Geometry: final body of the model. Coordinates: model frame, mm. A direction names the side the tool comes from. Give positions to 0.01 mm unless a question says otherwise; leave off trailing zeros. Order: outer loops, then holes, each group sorted by start corner. A loop starts at its lowest first (then second) coordinate and runs counter-clockwise, first axis right, second up. Notation, with made-up numbers: M 10.25,-24.5 L 15.25,-24.5 A35 ccw 15.25,11.5 Z; hole C 33,-27 d7. An arc over 180 degrees is marked long. Write item = value, one per line. Start each with the question number.
from build123d import *

# Parameters (mm, degrees)
IZIM1_R                     = 1.5
Y_KSEKLIK_EKSTR_ZYON1_DEPTH = 2
Y_KSEKLIK_EKSTR_ZYON2_START = -10
Y_KSEKLIK_EKSTR_ZYON2_DEPTH = 10
Y_KSEKLIK_EKSTR_ZYON3_START = -10
Y_KSEKLIK_EKSTR_ZYON3_DEPTH = 10
KAT_Y_D_N_T_R2_START        = 12.5
KAT_Y_D_N_T_R2_OUTLINE_W    = 10
KAT_Y_D_N_T_R2_OUTLINE_H    = 6
KAT_Y_D_N_T_R2_DEPTH        = 8
KAT_Y_D_N_T_R2_START_2      = 16.5
KAT_Y_D_N_T_R2_2_OUTLINE_W  = 10
KAT_Y_D_N_T_R2_2_OUTLINE_H  = 4
KAT_Y_D_N_T_R2_2_DEPTH      = 4
KENAR_START                 = -29.083147129
KENAR_EKME1_DEPTH           = 10
KENAR_START_2               = 19
KENAR_EKME1_2_DEPTH         = 10
PAH3_SIZE                   = 1


# Read off the part's stored shape, not the designer's step: Katıyı-Dönüştür2, Kenar Çekme1
with BuildPart() as part:
    # Çizim1 → Yükseklik-Ekstrüzyon1 (new body)
    with BuildSketch(Plane(origin=(0, 0, 0), x_dir=(1, 0, 0), z_dir=(0, 1, 0))):
        with BuildLine():
            Line((29, -12.5), (19, -12.5))
            Line((19, -12.5), (19, -6.464101615))
            Line((19, -6.464101615), (19, 3.5))
            ThreePointArc((19, 3.5), (18.121320344, 5.621320344), (16, 6.5))
            Line((16, 6.5), (-3.464101615, 6.5))
            Line((-3.464101615, 6.5), (-16.083147129, 6.5))
            ThreePointArc((-16.083147129, 6.5), (-18.204467472, 5.621320344), (-19.083147129, 3.5))
            Line((-19.083147129, 3.5), (-19.083147129, -6.464101615))
            Line((-19.083147129, -6.464101615), (-19.083147129, -12.5))
            Line((-19.083147129, -12.5), (-29.083147129, -12.5))
            Line((-29.083147129, -12.5), (-29.083147129, 13.5))
            ThreePointArc((-29.083147129, 13.5), (-28.204467472, 15.621320344), (-26.083147129, 16.5))
            Line((-26.083147129, 16.5), (26, 16.5))
            ThreePointArc((26, 16.5), (28.121320344, 15.621320344), (29, 13.5))
            Line((29, 13.5), (29, -12.5))
        make_face()
        with Locations(Location((-24.083147129, -3, 0), (0, 0, 270))):
            Circle(IZIM1_R, mode=Mode.SUBTRACT)
        with Locations(Location((0, 11.5, 0), (0, 0, 270))):
            Circle(IZIM1_R, mode=Mode.SUBTRACT)
        with Locations(Location((24, -3, 0), (0, 0, 270))):
            Circle(IZIM1_R, mode=Mode.SUBTRACT)
    extrude(amount=Y_KSEKLIK_EKSTR_ZYON1_DEPTH)

    # Çizim2 → Yükseklik-Ekstrüzyon2 (add)
    with BuildSketch(Plane(origin=(29, 0, 0), x_dir=(0, 0, -1), z_dir=(1, 0, 0)).offset(Y_KSEKLIK_EKSTR_ZYON2_START)):
        with BuildLine():
            Line((-14.767949192, 3), (-12.627016654, 3))
            ThreePointArc((-12.627016654, 3), (-18.949489743, 7.16227766), (-16.5, 0))
            Line((-16.5, 0), (-12.5, 0))
            Line((-12.5, 0), (-12.5, 2))
            Line((-12.5, 2), (-16.5, 2))
            ThreePointArc((-16.5, 2), (-17.5, 5.732050808), (-14.767949192, 3))
        make_face()
    extrude(amount=Y_KSEKLIK_EKSTR_ZYON2_DEPTH)

    # Çizim3 → Yükseklik-Ekstrüzyon3 (add)
    with BuildSketch(Plane(origin=(-19.083147129, 0, 0), x_dir=(0, 0, -1), z_dir=(1, 0, 0)).offset(Y_KSEKLIK_EKSTR_ZYON3_START)):
        with BuildLine():
            Line((-12.5, 2), (-16.5, 2))
            ThreePointArc((-16.5, 2), (-17.5, 5.732050808), (-14.767949192, 3))
            Line((-14.767949192, 3), (-12.627016654, 3))
            ThreePointArc((-12.627016654, 3), (-18.949489743, 7.16227766), (-16.5, 0))
            Line((-16.5, 0), (-12.5, 0))
            Line((-12.5, 0), (-12.5, 2))
        make_face()
    extrude(amount=Y_KSEKLIK_EKSTR_ZYON3_DEPTH)

    # Katıyı-Dönüştür2 outline → Katıyı-Dönüştür2 (cut)
    with BuildSketch(Plane.XY.offset(KAT_Y_D_N_T_R2_START)):
        with Locations((24, 6)):
            Rectangle(KAT_Y_D_N_T_R2_OUTLINE_W, KAT_Y_D_N_T_R2_OUTLINE_H)
        with Locations((-24.083147129, 6)):
            Rectangle(KAT_Y_D_N_T_R2_OUTLINE_W, KAT_Y_D_N_T_R2_OUTLINE_H)
    extrude(amount=KAT_Y_D_N_T_R2_DEPTH, mode=Mode.SUBTRACT)

    # Kat_y_-D_n_t_r2 2 outline → Kat_y_-D_n_t_r2 2 (cut)
    with BuildSketch(Plane.XY.offset(KAT_Y_D_N_T_R2_START_2)):
        with Locations((24, 1)):
            Rectangle(KAT_Y_D_N_T_R2_2_OUTLINE_W, KAT_Y_D_N_T_R2_2_OUTLINE_H)
        with Locations((-24.083147129, 1)):
            Rectangle(KAT_Y_D_N_T_R2_2_OUTLINE_W, KAT_Y_D_N_T_R2_2_OUTLINE_H)
    extrude(amount=KAT_Y_D_N_T_R2_2_DEPTH, mode=Mode.SUBTRACT)

    # Kenar Çekme1 outline → Kenar Çekme1 (add)
    with BuildSketch(Plane.YZ.offset(KENAR_START)):
        with BuildLine():
            Line((3.448725288, 14.577476608), (2.897450577, 12.654953216))
            ThreePointArc((2.897450577, 12.654953216), (7.19454204, 18.907260093), (0, 16.5))
            Line((0, 16.5), (2, 16.5))
            ThreePointArc((2, 16.5), (5.59727102, 17.703630046), (3.448725288, 14.577476608))
        make_face()
    extrude(amount=KENAR_EKME1_DEPTH)

    # Kenar _ekme1 2 outline → Kenar _ekme1 2 (add)
    with BuildSketch(Plane.YZ.offset(KENAR_START_2)):
        with BuildLine():
            Line((3.448725288, 14.577476608), (2.897450577, 12.654953216))
            ThreePointArc((2.897450577, 12.654953216), (7.19454204, 18.907260093), (0, 16.5))
            Line((0, 16.5), (2, 16.5))
            ThreePointArc((2, 16.5), (5.59727102, 17.703630046), (3.448725288, 14.577476608))
        make_face()
    extrude(amount=KENAR_EKME1_2_DEPTH)

    # Pah3
    pah3_edges = [part.edges().sort_by_distance(p)[0] for p in [
        (24, 2, 1.5),
        (-24.083147129, 2, 1.5),
        (0, 2, -13),
    ]]
    chamfer(pah3_edges, length=PAH3_SIZE)


solid = part.part
1) Cut plane A-A (x = 0). Return loops of the section in (y, z).
2) Pin query (flat end, axial travel): pin 1 Ø1 at (x, y) = (2, 0.5) entering from +Z. Return the tip coordinate at first contact, or that it passes through.
3) Access query for faces 5 (the cylindrical face through (0.07, 0.49, -13)), 6 (the flat face through (0, 1, -6.5)), 7 (the flat face through (-24.153, 3.177, 13.63)). Directions: +Z, -Z, +X, -X, +Y, -Y. A direction counts if a zero-diameter tool reaches every point of the face in a straight line with its end or side. Return the directions, or none.
4) Cut plane C-C (z = 3). Return loops of the section in (x, y).
5) Cut plane D-D (y = 7.25). Return loops of the section in (x, z).
6) Ray query, L1, parallel to X at y = 0.7, z = 3; L2, parallel to X at y = 6.75, z = 14; L3, parallel to Y at x = -3, z = -12. Return the intervals inside material, ascending.
7) Draft query along Z for faces 1 (the cylindrical face through (-28.228, 0.986, -15.598)), 2 (the cylindrical face through (25.487, 0.493, 2.805)), 3 (the cylindrical face through (-25.547, 0.493, 2.675)), 4 (the flat face through (0, 0, -7)). Return one class per face: pulls with the +Z half, pulls with the -Z half, needs draft (parallel to the pull), parting line crosses it, or undercut.
8) Cut plane B-B (z = -11.5). Return loops of the section in (x, y), plus the area to 3 significant figures.
Reply:
q1.outline = M 0,-16.5 L 2,-16.5 L 2,-14 L 1,-13 L 0,-13 Z; M 0,-10 L 1,-10 L 2,-9 L 2,-6.5 L 0,-6.5 Z
q2.pin_1 = -6.5
q3.face_5 = +Y, -Y
q3.face_6 = +Z, +Y, -Y
q3.face_7 = +X, -X
q4.outline = M -29.08,0 L -25.58,0 L -25.58,1 L -26.58,2 L -29.08,2 Z; M -22.58,0 L -19.08,0 L -19.08,2 L -21.58,2 L -22.58,1 Z; M 19,0 L 22.5,0 L 22.5,1 L 21.5,2 L 19,2 Z; M 25.5,0 L 29,0 L 29,2 L 26.5,2 L 25.5,1 Z
q5.outline = M -29.08,14.17 L -19.08,14.17 L -19.08,18.83 L -29.08,18.83 Z; M 19,14.17 L 29,14.17 L 29,18.83 L 19,18.83 Z
q6.L1 = -29.08 to -25.58, -22.58 to -19.08, 19 to 22.5, 25.5 to 29
q6.L2 = -29.08 to -19.08, 19 to 29
q6.L3 = 0 to 2
q7.face_1 = pulls with the -Z half
q7.face_2 = undercut
q7.face_3 = undercut
q7.face_4 = needs draft
q8.outline = M -29.08,0 L -1.5,0 L -1.5,1 L -2.5,2 L -29.08,2 Z; M 1.5,0 L 29,0 L 29,2 L 2.5,2 L 1.5,1 Z
q8.area = 109 mm²
